from build123d import *

# Parameters (mm, degrees)
F0_W     = 255
F0_H     = 150
F0_R     = 3
F0_R_2   = 6
F1_DEPTH = 6


with BuildPart() as f1:
    # F0 (on Front) → F1 (new body)
    with BuildSketch(Plane.XZ):
        with Locations((67.5, -15)):
            Rectangle(F0_W, F0_H)
        with Locations((-50, -80)):
            Circle(F0_R, mode=Mode.SUBTRACT)
        with Locations((55, -60)):
            Circle(F0_R, mode=Mode.SUBTRACT)
        with Locations((185, -80)):
            Circle(F0_R, mode=Mode.SUBTRACT)
        with Locations((165, -60)):
            Circle(F0_R, mode=Mode.SUBTRACT)
        Circle(F0_R, mode=Mode.SUBTRACT)
        with Locations((55, 0)):
            Circle(F0_R_2, mode=Mode.SUBTRACT)
        with Locations((-50, 50)):
            Circle(F0_R, mode=Mode.SUBTRACT)
        with Locations((122.5, 0)):
            Circle(F0_R, mode=Mode.SUBTRACT)
        with Locations((185, 50)):
            Circle(F0_R, mode=Mode.SUBTRACT)
    extrude(amount=F1_DEPTH)


solid = f1.part
For this review, take the finished solid that the model builds, in its own axes (mm). Give positions to 0.01 mm unless a question says otherwise; leave off trailing zeros. Loops run counter-clockwise (first coordinate to the right, second up) from the corner with the lowest first, then second, coordinate; pieces in that order, holes last. Notation, with made-up numbers: (-17, 6.5) - (34, 6.5) arc R18 cw to (34, 17.5) - close; hole circle Ø11 at (79, -34.75). An arc over 180 degrees is marked (long way). Write each question's results on one line, items separated by ' | '.
(1) Take a section at A-A (x = 165). Give the boundary of the cut face in (y, z).
Conclusion:
outline: (-6, -90) - (0, -90) - (0, -63) - (-6, -63) - close; (-6, -57) - (0, -57) - (0, 60) - (-6, 60) - close
(2) Take a section at D-D (z = 0). Give the boundary of the cut face in (x, y).
Conclusion:
outline: (-60, -6) - (-3, -6) - (-3, 0) - (-60, 0) - close; (3, -6) - (49, -6) - (49, 0) - (3, 0) - close; (61, -6) - (119.5, -6) - (119.5, 0) - (61, 0) - close; (125.5, -6) - (195, -6) - (195, 0) - (125.5, 0) - close
(3) Take a section at C-C (x = 55). Give the boundary of the cut face in (y, z).
Conclusion:
outline: (-6, -90) - (0, -90) - (0, -63) - (-6, -63) - close; (-6, -57) - (0, -57) - (0, -6) - (-6, -6) - close; (-6, 6) - (0, 6) - (0, 60) - (-6, 60) - close
(4) Draft analysis for pull direction X (two halves, no side actions). For faces 1 (the cylindrical face through (49, -3, 0)), 2 (the cylindrical face through (-52.21, -2.96, 52.03)), 3 (the flat face through (66, -3, -90)), 4 (the flat face through (-60, -3, -16)), state which applies: +X half, -X half, draft (parallel to the pull), parting line (faces both ways), or undercut.
Conclusion:
face 1: undercut | face 2: undercut | face 3: draft | face 4: -X half
(5) For line 1 along Z through (x, y) = (185, -1.95); line 2 along X through (y, z) = (-2.7, -62); line 3 along Z through (x, y) = (165, -1.55), list the stretches that pass through material, from the lowest coordinate up.
Conclusion:
line 1: -90 to -83, -77 to 47, 53 to 60 | line 2: -60 to 52.76, 57.24 to 162.76, 167.24 to 195 | line 3: -90 to -63, -57 to 60
(6) Take a section at B-B (z = -80). Give the boundary of the cut face in (x, y), then the cut area to 3 significant figures.
Conclusion:
outline: (-60, -6) - (-53, -6) - (-53, 0) - (-60, 0) - close; (-47, -6) - (182, -6) - (182, 0) - (-47, 0) - close; (188, -6) - (195, -6) - (195, 0) - (188, 0) - close | area: 1,460 mm^2
